For this review, use the dimensioned drawing (mm, ordinates from the lowest corner) and the shaded views. Coordinates: 2 decimals unless noted, no trailing zeros. Loops run counter-clockwise (first coordinate to the right, second up) from the corner with the lowest first, then second, coordinate; pieces in that order, holes last. Notation, with made-up numbers: (-12.75, 43.5) -> (28.25, 43.5) arc R24 cw to (28.25, 53.5) -> close; hole circle Ø1 at (56, 85.25). An arc over 180 degrees is marked (long way). Answer as a JSON object with one key per item and string values.
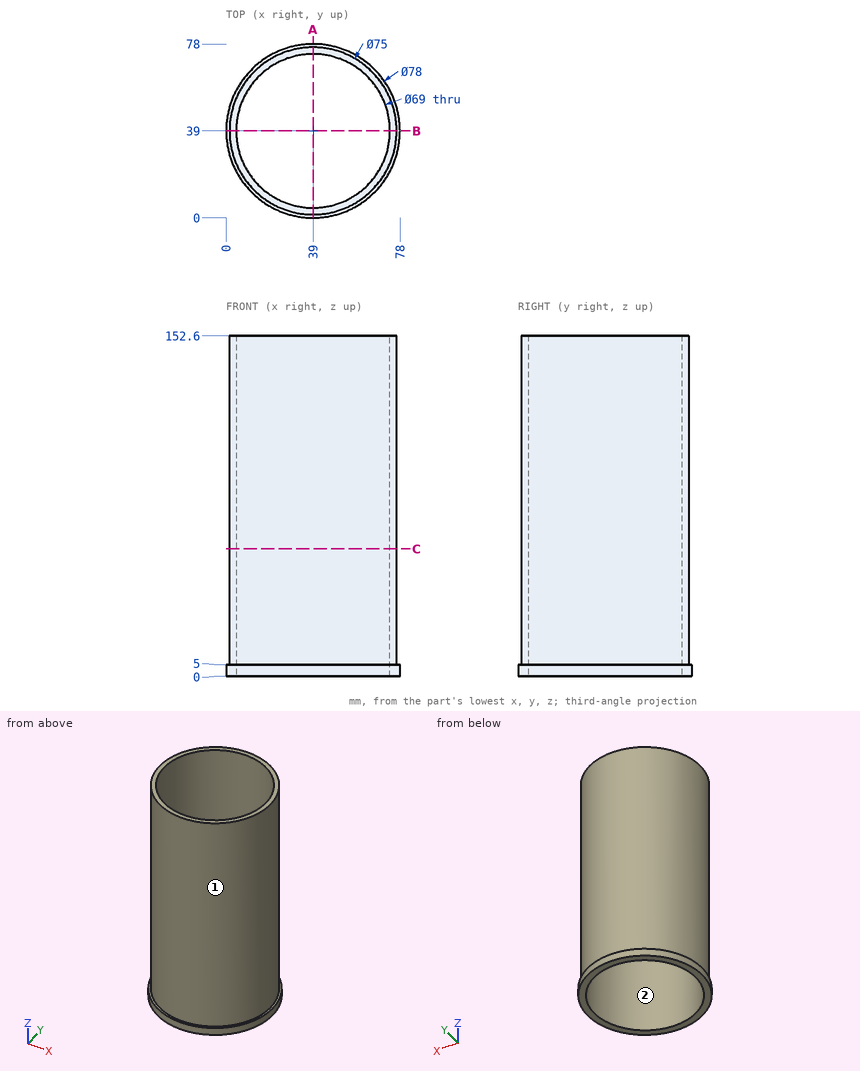
1) The part is to be moulded in two halves that separate along X. For the marked faces 1 and 2, say which applies: pulls with the +X half, pulls with the -X half, needs draft (parallel to the pull), parting line crosses it, or undercut.
Completed:
{"face 1": "parting line crosses it", "face 2": "undercut"}
2) Add section A-A, the plane x = 39. Give the boundary of the cut face in (y, z), and give its area (3 significant figures).
Completed:
{"outline": "(0, 0) -> (4.5, 0) -> (4.5, 152.6) -> (1.5, 152.6) -> (1.5, 5) -> (0, 5) -> close; (73.5, 0) -> (78, 0) -> (78, 5) -> (76.5, 5) -> (76.5, 152.6) -> (73.5, 152.6) -> close", "area": "931 mm²"}
3) Clearance check with flat-ended pins moving along their axes: pin 1 Ø8 at (x, z) = (16, 26) entering from -Y; pin 2 Ø6 at (y, z) = (51.5, 102.5) entering from -X; pin 3 Ø8 at (y, z) = (38, 122) entering from -X. State where each tip first meets the part, or that it passes through.
Completed:
{"pin 1": "y = 6.67", "pin 2": "x = 2.72", "pin 3": "x = 1.5"}
4) Add section C-C, the plane z = 57. Give the boundary of the cut face in (x, y), and give its area (3 significant figures).
Completed:
{"outline": "circle Ø75 at (39, 39); hole circle Ø69 at (39, 39)", "area": "679 mm²"}
5) Wall thickness on probe 1 along Y at (x, z) = (40.5, 54.5); probe 2 along X at (y, z) = (13, 27); probe 3 along X at (y, z) = (29, 135): over which ranges is each line inside the solid? List them lowest first.
Completed:
{"probe 1": "1.53 to 4.53, 73.47 to 76.47", "probe 2": "11.98 to 16.32, 61.68 to 66.02", "probe 3": "2.86 to 5.98, 72.02 to 75.14"}
